Source: CAD feature listing. Evaluate the final solid. Frame: model axes, mm. Face numbers are marked on the shaded views. A direction names the side the tool comes from. Coordinates: 2 decimals unless noted, no trailing zeros. Write each loop counter-clockwise with the first axis right and the second up, starting at its lowest first coordinate (ties: lowest second). Pieces come first, ordered by that corner, then holes. Notation, with made-up numbers: M 48,15 L 89,15 A24 ccw 89,29 Z; hole C 3.25,10 d1. An arc over 180 degrees is marked long. Answer as CSV lines item,"result". Start each with the question number.
1. Contact query for flat-ended pins moving along their axis: pin 1 Ø3 at (x, y) = (-3, 13.5) entering from +Z; pin 2 Ø6 at (x, z) = (4, 10) entering from +Y. Output: stop coordinate, or through.
2. Mould query, pull axis X, two halves, no side actions, for the marked faces 1, 2 and 3. Classes: pulls with the +X half, pulls with the -X half, needs draft (parallel to the pull), parting line crosses it, or undercut.
3. Section D-D on z = 7.25. Return the cut outline in (x, y), plus the area to 3 significant figures.
4. Section C-C on y = 5. Return the cut outline in (x, z), plus the area to 3 significant figures.
5. Section B-B on z = 11.25. Return the cut outline in (x, y).
6. Line query: probe 1 along Y at (x, z) = (3.5, 8); probe 2 along X at (y, z) = (3, 9); probe 3 along X at (y, z) = (4, 7). Output: solid intervals per line, ascending. Write a range as [from, to].
7. Section A-A on x = 3.4. Return the cut outline in (y, z).
8. Reachability of the marked faces 4, 5, 6 and 7 from +Z, -Z, +X, -X, +Y, -Y: full face, straight path, thin tool, end or side. Return the list, or none.
```python
from build123d import *

# Parameters (mm, degrees)
F1_DEPTH    = 12
F0_W        = 8.5
F0_H        = 10
F2_DEPTH    = 2
F4_D        = 2.8
F6_W        = 1
F6_H        = 6
F7_DEPTH    = 2
F8_T1_DEPTH = 3
F8_T3_DEPTH = 3


# Not quite as in the source:
# - a fillet or chamfer that OpenCascade refuses, or shapes differently, is made with other operations: its cross-section is extruded or revolved along the edge and cut away or added


with BuildPart() as f1:
    # F0 (on Top) → F1 (new body)
    with BuildSketch(Plane.XY):
        with BuildLine():
            Line((0, 2), (0, 0))
            Line((0, 0), (5.9, 0))
            Line((5.9, 0), (5.9, 6))
            Line((5.9, 6), (-2.6, 6))
            Line((-2.6, 6), (-2.6, 4.6))
            ThreePointArc((-2.6, 4.6), (-0.7615223689, 3.8384776311), (0, 2))
        make_face()
    extrude(amount=F1_DEPTH)

    # F0 (on Top) → F2 (join)
    with BuildSketch(Plane.XY):
        with Locations((1.65, 11)):
            Rectangle(F0_W, F0_H)
    extrude(amount=F2_DEPTH)

    # F4 (through all)
    with Locations(Plane.XY.offset(12)):
        with Locations((3.4, 3)):
            Hole(F4_D / 2)

    # F5: F1 across face


with BuildPart() as f1_1:
    add(f1.part)
    add(f1.part.mirror(Plane(origin=(-2.6, 8.397826087, 3.2826086957), x_dir=(0, -1, 0), z_dir=(-1, 0, 0))))

    # F6 (on face) → F7 (join)
    with BuildSketch(Plane.XY.offset(12)):
        with Locations((-10.6, 3)):
            Rectangle(F6_W, F6_H)
        with BuildLine():
            Line((1.9, 6), (-7.1, 6))
            Line((-7.1, 6), (-7.1, 0))
            Line((-7.1, 0), (-5.2, 0))
            Line((-5.2, 0), (-5.2, 2))
            ThreePointArc((-5.2, 2), (-2.6, 4.6), (0, 2))
            Line((0, 2), (0, 0))
            Line((0, 0), (1.9, 0))
            Line((1.9, 0), (1.9, 6))
        make_face()
        with Locations((5.4, 3)):
            Rectangle(F6_W, F6_H)
    extrude(amount=F7_DEPTH)

    # F8: chamfer of 2 on 2 edges, made by hand

    # F8_s2 → F8_t1 (cut)
    with BuildSketch(Plane.YZ.offset(-10.1)):
        Polygon((2, 12), (0, 10), (0, 12), align=None)
    extrude(amount=F8_T1_DEPTH, mode=Mode.SUBTRACT)

    # F8_s4 → F8_t3 (cut)
    with BuildSketch(Plane.YZ.offset(1.9)):
        Polygon((2, 12), (0, 10), (0, 12), align=None)
    extrude(amount=F8_T3_DEPTH, mode=Mode.SUBTRACT)


solid = f1_1.part
```
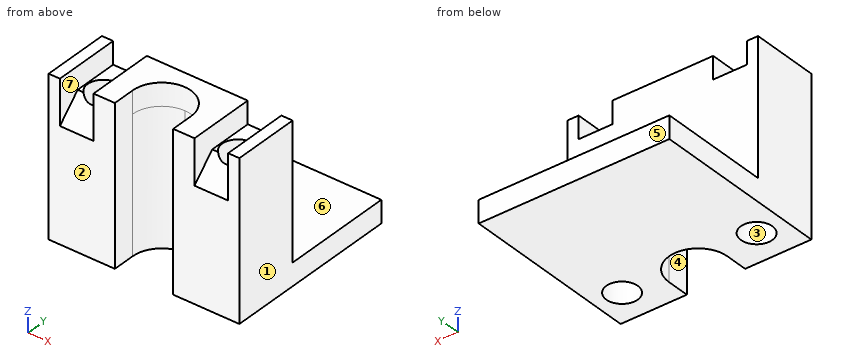
Values:
1,pin 1,"z = 2"
1,pin 2,"y = 6"
2,face 1,"pulls with the +X half"
2,face 2,"needs draft"
2,face 3,"undercut"
3,outline,"M -11.1,0 L -5.2,0 L -5.2,2 A2.6 cw 0,2 L 0,0 L 5.9,0 L 5.9,6 L -11.1,6 Z; hole C -8.6,3 d2.8; hole C 3.4,3 d2.8"
3,area,"68.7 mm²"
4,outline,"M -11.1,0 L 5.9,0 L 5.9,14 L 4.9,14 L 4.9,12 L 1.9,12 L 1.9,14 L -7.1,14 L -7.1,12 L -10.1,12 L -10.1,14 L -11.1,14 Z"
4,area,"226 mm²"
5,outline,"M -11.1,0 L -10.1,0 L -10.1,1.25 L -7.1,1.25 L -7.1,0 L -5.2,0 L -5.2,2 A2.6 cw 0,2 L 0,0 L 1.9,0 L 1.9,1.25 L 4.9,1.25 L 4.9,0 L 5.9,0 L 5.9,6 L -11.1,6 Z; hole C -8.6,3 d2.8; hole C 3.4,3 d2.8"
6,probe 1,"[0, 1.6], [4.4, 6]"
6,probe 2,"[-11.1, -10], [-7.2, -5], [-0.2, 2], [4.8, 5.9]"
6,probe 3,"[-11.1, -9.58], [-7.62, -4.26], [-0.94, 2.42], [4.38, 5.9]"
7,outline,"M 0,0 L 1.6,0 L 1.6,11.6 L 0,10 Z; M 4.4,0 L 16,0 L 16,2 L 6,2 L 6,12 L 4.4,12 Z"
8,face 4,"+Z, -Z, -Y"
8,face 5,"+Z, -Z, +X, -X, +Y"
8,face 6,"+Z, +X, -X, +Y"
8,face 7,"+Z, -Y"
